Verification items for this drawing (mm, ordinates from the low corner). Coordinates: 2 decimals unless noted, no trailing zeros. Order: outer loops, then holes, each group sorted by start corner. A loop starts at its lowest first (then second) coordinate and runs counter-clockwise, first axis right, second up. Notation, with made-up numbers: M 18,18 L 31,18 A23 cw 31,49 Z; hole C -4,-20 d11. An arc over 180 degrees is marked long. Write item = value, one per line.
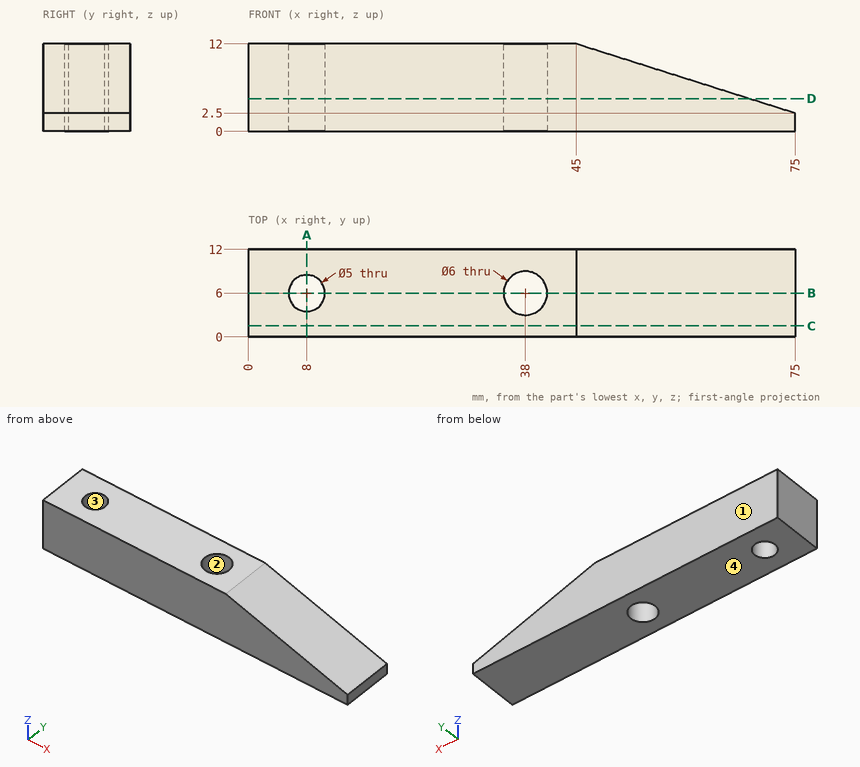
Item 1: Release check for a two-part mould opening along Y. For the marked faces 1, 2, 3 and 4 record: pulls with the +Y half, pulls with the -Y half, needs draft (parallel to the pull), parting line crosses it, or undercut.
Report:
face_1 = pulls with the +Y half
face_2 = undercut
face_3 = undercut
face_4 = needs draft
Item 2: Sectioned sample at A-A, the plane x = 8. Enter the section's corners in (y, z).
Report:
outline = M 0,0 L 3.5,0 L 3.5,12 L 0,12 Z; M 8.5,0 L 12,0 L 12,12 L 8.5,12 Z
Item 3: Scan lines: L1, parallel to Y at x = 38, z = 4; L2, parallel to Y at x = 8, z = 6.5; L3, parallel to X at y = 3.75, z = 1.5. Record each from-to range of solid material in increasing order. Write a range as from..to.
Report:
L1 = 0..3, 9..12
L2 = 0..3.5, 8.5..12
L3 = 0..6.91, 9.09..36.02, 39.98..75
Item 4: Sectioned sample at D-D, the plane z = 4.5. Enter the section's corners in (x, y), then the cut area to 3 significant figures.
Report:
outline = M 0,0 L 68.68,0 L 68.68,12 L 0,12 Z; hole C 8,6 d5; hole C 38,6 d6
area = 776 mm^2
Item 5: Sectioned sample at B-B, the plane y = 6. Enter the section's corners in (x, z), then the cut area to 4 significant figures.
Report:
outline = M 0,0 L 5.5,0 L 5.5,12 L 0,12 Z; M 10.5,0 L 35,0 L 35,12 L 10.5,12 Z; M 41,0 L 75,0 L 75,2.5 L 45,12 L 41,12 Z
area = 625.5 mm^2
Item 6: Sectioned sample at C-C, the plane y = 1.5. Enter the section's corners in (x, z).
Report:
outline = M 0,0 L 75,0 L 75,2.5 L 45,12 L 0,12 Z
Item 7: Gauge pin test, flat end, axial feed: pin 1 (1.5 mm diameter, centred on x = 65.5, y = 4, fed in from +Z). Record the tip position at first contact, or that the pin passes through.
Report:
pin_1 = 5.75
